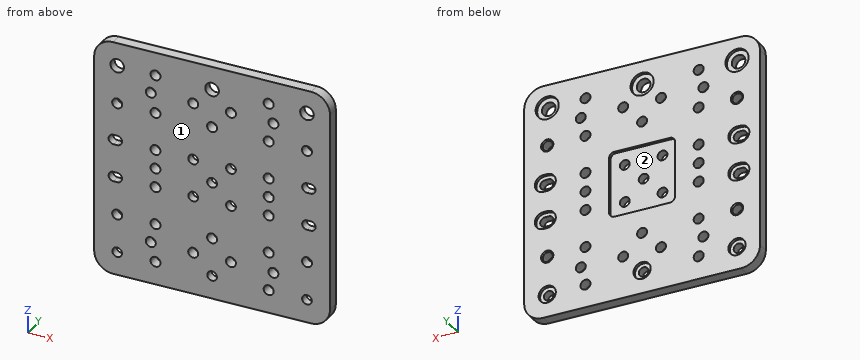
```python
from build123d import *

# Parameters (mm, degrees)
SKETCH1_W                        = 125
SKETCH1_H                        = 125
BOSS_EXTRUDE1_DEPTH              = 6
CBORE_FOR_M6_5_SHSS1_D           = 7.2
CBORE_FOR_M6_5_SHSS1_CBORE_D     = 12.25
CBORE_FOR_M6_5_SHSS1_CBORE_DEPTH = 1.6
HOLE1_D                          = 5.1
HOLE1_DEPTH                      = 6
HOLE1_CBORE_D                    = 9.14
HOLE1_CBORE_DEPTH                = 1.6
HOLE1_TIP                        = 1.532194579
F_5_3_5_3_DIAMETER_HOLE1_D       = 5.3
F_5_3_5_3_DIAMETER_HOLE2_D       = 5.3
CUT_EXTRUDE1_DEPTH               = 1.6
CUT_EXTRUDE2_DEPTH               = 89.497796583
SKETCH16_W                       = 35
SKETCH16_H                       = 35
CUT_EXTRUDE3_DEPTH               = 1.6
F_5_2_5_2_DIAMETER_HOLE1_D       = 5.2
FILLET1_R                        = 10
FILLET2_R                        = 2.8
F_5_3_5_3_DIAMETER_HOLE3_D       = 5.3
CHAMFER1_SIZE                    = 0.6


with BuildPart() as part:
    # Sketch1 → Boss-Extrude1 (new body)
    with BuildSketch(Plane(origin=(0, 0, 0), x_dir=(1, 0, 0), z_dir=(0, 1, 0))):
        Rectangle(SKETCH1_W, SKETCH1_H)
    extrude(amount=BOSS_EXTRUDE1_DEPTH)

    # CBORE for M6.5 SHSS1 (through all)
    with Locations(Plane(origin=(0, 6, 0), x_dir=(1, 0, 0), z_dir=(0, 1, 0))):
        with Locations((-50.3, -50.3), (0, -50.3), (50.3, -50.3)):
            CounterBoreHole(CBORE_FOR_M6_5_SHSS1_D / 2, CBORE_FOR_M6_5_SHSS1_CBORE_D / 2, CBORE_FOR_M6_5_SHSS1_CBORE_DEPTH)

    # Hole1
    with Locations(Plane(origin=(0, 6, 0), x_dir=(1, 0, 0), z_dir=(0, 1, 0))):
        with Locations((-50.3, 50.3), (0, 50.3), (50.3, 50.3)):
            CounterBoreHole(HOLE1_D / 2, HOLE1_CBORE_D / 2, HOLE1_CBORE_DEPTH, depth=HOLE1_DEPTH)
            with Locations((0, 0, -(HOLE1_DEPTH + HOLE1_TIP / 2))):  # 118° drill point
                Cone(0, HOLE1_D / 2, HOLE1_TIP, mode=Mode.SUBTRACT)

    # Ø5.3 (5.3) Diameter Hole1 (through all)
    with Locations(Plane(origin=(0, 6, 0), x_dir=(1, 0, 0), z_dir=(0, 1, 0))):
        with Locations((-30, 50.3), (-32.5, 40.3), (-30, 30), (-10, 40.3), (0, 30), (-30, 10), (-30, 0)):
            Hole(F_5_3_5_3_DIAMETER_HOLE1_D / 2)

    # Ø5.3 (5.3) Diameter Hole2 (through all)
    with Locations(Plane(origin=(0, 6, 0), x_dir=(1, 0, 0), z_dir=(0, 1, 0))):
        with Locations((10, 40.3), (30, 50.3), (32.5, 40.3), (30, 30), (30, 10), (30, 0), (30, -10), (-30, -10), (-30, -30), (0, -30), (30, -30), (10, -40.3), (-10, -40.3), (-32.5, -40.3), (32.5, -40.3), (30, -50.3), (-30, -50.3)):
            Hole(F_5_3_5_3_DIAMETER_HOLE2_D / 2)

    # Sketch13 → Cut-Extrude1 (cut)
    with BuildSketch(Plane(origin=(0, 6, 0), x_dir=(1, 0, 0), z_dir=(0, 1, 0))):
        with BuildLine():
            Line((52.3, 5.43), (50.3, 5.43))
            ThreePointArc((50.3, 5.43), (45.73, 10), (50.3, 14.57))
            Line((50.3, 14.57), (52.3, 14.57))
            ThreePointArc((52.3, 14.57), (56.87, 10), (52.3, 5.43))
        make_face()
        with BuildLine():
            Line((-52.3, 14.57), (-50.3, 14.57))
            ThreePointArc((-50.3, 14.57), (-45.73, 10), (-50.3, 5.43))
            Line((-50.3, 5.43), (-52.3, 5.43))
            ThreePointArc((-52.3, 5.43), (-56.87, 10), (-52.3, 14.57))
        make_face()
        with BuildLine():
            Line((-52.3, -5.43), (-50.3, -5.43))
            ThreePointArc((-50.3, -5.43), (-45.73, -10), (-50.3, -14.57))
            Line((-50.3, -14.57), (-52.3, -14.57))
            ThreePointArc((-52.3, -14.57), (-56.87, -10), (-52.3, -5.43))
        make_face()
        with BuildLine():
            Line((52.3, -14.57), (50.3, -14.57))
            ThreePointArc((50.3, -14.57), (45.73, -10), (50.3, -5.43))
            Line((50.3, -5.43), (52.3, -5.43))
            ThreePointArc((52.3, -5.43), (56.87, -10), (52.3, -14.57))
        make_face()
    extrude(amount=-CUT_EXTRUDE1_DEPTH, mode=Mode.SUBTRACT)

    # Sketch15 → Cut-Extrude2 (cut, through all)
    with BuildSketch(Plane(origin=(0, 4.4, 0), x_dir=(1, 0, 0), z_dir=(0, 1, 0))):
        with BuildLine():
            Line((52.3, 7.45), (50.3, 7.45))
            ThreePointArc((50.3, 7.45), (47.75, 10), (50.3, 12.55))
            Line((50.3, 12.55), (52.3, 12.55))
            ThreePointArc((52.3, 12.55), (54.85, 10), (52.3, 7.45))
        make_face()
        with BuildLine():
            Line((-52.3, 12.55), (-50.3, 12.55))
            ThreePointArc((-50.3, 12.55), (-47.75, 10), (-50.3, 7.45))
            Line((-50.3, 7.45), (-52.3, 7.45))
            ThreePointArc((-52.3, 7.45), (-54.85, 10), (-52.3, 12.55))
        make_face()
        with BuildLine():
            Line((-52.3, -7.45), (-50.3, -7.45))
            ThreePointArc((-50.3, -7.45), (-47.75, -10), (-50.3, -12.55))
            Line((-50.3, -12.55), (-52.3, -12.55))
            ThreePointArc((-52.3, -12.55), (-54.85, -10), (-52.3, -7.45))
        make_face()
        with BuildLine():
            Line((50.3, -7.45), (52.3, -7.45))
            ThreePointArc((52.3, -7.45), (54.85, -10), (52.3, -12.55))
            Line((52.3, -12.55), (50.3, -12.55))
            ThreePointArc((50.3, -12.55), (47.75, -10), (50.3, -7.45))
        make_face()
    extrude(amount=-CUT_EXTRUDE2_DEPTH, mode=Mode.SUBTRACT)

    # Sketch16 → Cut-Extrude3 (cut)
    with BuildSketch(Plane(origin=(0, 6, 0), x_dir=(1, 0, 0), z_dir=(0, 1, 0))):
        Rectangle(SKETCH16_W, SKETCH16_H)
    extrude(amount=-CUT_EXTRUDE3_DEPTH, mode=Mode.SUBTRACT)

    # Ø5.2 (5.2) Diameter Hole1 (through all)
    with Locations(Plane(origin=(0, 4.4, 0), x_dir=(1, 0, 0), z_dir=(0, 1, 0))):
        with Locations((-10, 10), (0, 0), (10, 10), (10, -10), (-10, -10)):
            Hole(F_5_2_5_2_DIAMETER_HOLE1_D / 2)

    # Fillet1
    fillet1_edges = [part.edges().sort_by_distance(p)[0] for p in [
        (62.5, 3, 62.5),
        (-62.5, 3, 62.5),
        (-62.5, 3, -62.5),
        (62.5, 3, -62.5),
    ]]
    fillet(fillet1_edges, radius=FILLET1_R)

    # Fillet2
    fillet2_edges = [part.edges().sort_by_distance(p)[0] for p in [
        (17.5, 5.2, -17.5),
        (17.5, 5.2, 17.5),
        (-17.5, 5.2, 17.5),
        (-17.5, 5.2, -17.5),
    ]]
    fillet(fillet2_edges, radius=FILLET2_R)

    # Ø5.3 (5.3) Diameter Hole3 (through all)
    with Locations(Plane(origin=(0, 6, 0), x_dir=(1, 0, 0), z_dir=(0, 1, 0))):
        with Locations((-50.3, 30), (50.3, 30), (50.3, -30), (-50.3, -30)):
            Hole(F_5_3_5_3_DIAMETER_HOLE3_D / 2)

    # Chamfer1
    chamfer1_edges = [part.edges().sort_by_distance(p)[0] for p in [
        (-47.65, 6, 30),
        (52.95, 6, 30),
        (52.95, 6, -30),
        (-47.65, 6, -30),
    ]]
    chamfer(chamfer1_edges, length=CHAMFER1_SIZE)


solid = part.part
```
Design review of the part built by this model. Coordinates are the model's own, in mm. Face numbers are marked on the shaded views. Round coordinates to 2 decimals unless told otherwise and drop trailing zeros. Order: outer loops, then holes, each group sorted by start corner. A loop starts at its lowest first (then second) coordinate and runs counter-clockwise, first axis right, second up. Notation, with made-up numbers: (-18.5, 19) - (8.5, 19) arc R15 cw to (8.5, 24) - close; hole circle Ø2 at (89.5, -9.5). An arc over 180 degrees is marked (long way). Return JSON: item names as keys, results as strings.
Q1. For pin 1 Ø1.5 at (x, z) = (-35, -25.5) entering from -Y, flat-tipped, find the tip position at first contact; note if it passes through.
Computed values:
{"pin 1": "stops at y = 0"}
Q2. Consider section A-A on z = -30. Write out the cut boundary in (x, y), plus the area to 3 significant figures.
Computed values:
{"outline": "(-62.5, 0) - (-52.95, 0) - (-52.95, 5.4) - (-53.55, 6) - (-62.5, 6) - close; (-47.65, 0) - (-32.65, 0) - (-32.65, 6) - (-47.05, 6) - (-47.65, 5.4) - close; (-27.35, 0) - (-2.65, 0) - (-2.65, 6) - (-27.35, 6) - close; (2.65, 0) - (27.35, 0) - (27.35, 6) - (2.65, 6) - close; (32.65, 0) - (47.65, 0) - (47.65, 5.4) - (47.05, 6) - (32.65, 6) - close; (52.95, 0) - (62.5, 0) - (62.5, 6) - (53.55, 6) - (52.95, 5.4) - close", "area": "590 mm2"}
Q3. Consider section C-C on y = 1.9. Give the number of separate pieces and of enclosed holes in the cut face, plus the area to 3 significant figures.
Computed values:
{"separate pieces": "1", "enclosed holes": "43", "area": "14,500 mm2"}
Q4. The part is to be moulded in two halves that separate along Z. For the marked faces 1 and 2, say which applies: pulls with the +Z half, pulls with the -Z half, needs draft (parallel to the pull), parting line crosses it, or undercut.
Computed values:
{"face 1": "needs draft", "face 2": "undercut"}
Q5. Wall thickness on L1, parallel to X at y = 1.85, z = -30; L2, parallel to Z at x = 10, y = 3.35; L3, parallel to X at y = 3.8, z = -40.3: over which ranges is each line inside the solid? List them lowest first. Write a range as [from, to].
Computed values:
{"L1": "x = [-62.5, -52.95], [-47.65, -32.65], [-27.35, -2.65], [2.65, 27.35], [32.65, 47.65], [52.95, 62.5]", "L2": "z = [-62.5, -42.95], [-37.65, -12.6], [-7.4, 7.4], [12.6, 37.65], [42.95, 62.5]", "L3": "x = [-62.5, -35.15], [-29.85, -12.65], [-7.35, 7.35], [12.65, 29.85], [35.15, 62.5]"}
Q6. Consider section B-B on x = 10. Write out the cut boundary in (y, z).
Computed values:
{"outline": "(0, -62.5) - (6, -62.5) - (6, -42.95) - (0, -42.95) - close; (0, -37.65) - (6, -37.65) - (6, -17.5) - (4.4, -17.5) - (4.4, -12.6) - (0, -12.6) - close; (0, -7.4) - (4.4, -7.4) - (4.4, 7.4) - (0, 7.4) - close; (0, 12.6) - (4.4, 12.6) - (4.4, 17.5) - (6, 17.5) - (6, 37.65) - (0, 37.65) - close; (0, 42.95) - (6, 42.95) - (6, 62.5) - (0, 62.5) - close"}
